from build123d import *

# Parameters (mm, degrees)
F0_W          = 17
F0_H          = 4
F1_DEPTH      = 50
F0_R          = 1.75
F0_R_2        = 11.5
F0_W_2        = 13
F2_DEPTH      = 3
F4_DEPTH      = 5
F4_DEPTH_BACK = 50
F6_DEPTH      = 3


with BuildPart() as f1:
    # F0 (on Top) → F1 (new body)
    with BuildSketch(Plane.XY):
        Polygon((-21.5, -21.5), (-21.5, 21.5), (-24.5, 21.5), (-24.5, -25.5), (-21.5, -25.5), align=None)
        Polygon((24.5, -25.5), (21.5, -25.5), (8.5, -25.5), (-8.5, -25.5), (-21.5, -25.5), (-24.5, -25.5), (-24.5, -28.5), (24.5, -28.5), align=None)
        Polygon((24.5, 21.5), (21.5, 21.5), (21.5, -21.5), (21.5, -25.5), (24.5, -25.5), align=None)
        with Locations((0, -23.5)):
            Rectangle(F0_W, F0_H)
    extrude(amount=F1_DEPTH)

    # F0 (on Top) → F2 (join)
    with BuildSketch(Plane.XY):
        Polygon((21.5, -21.5), (21.5, 21.5), (-21.5, 21.5), (-21.5, -21.5), (-8.5, -21.5), (8.5, -21.5), align=None)
        with Locations((-15.5, -15.5)):
            Circle(F0_R, mode=Mode.SUBTRACT)
        with Locations((15.5, -15.5)):
            Circle(F0_R, mode=Mode.SUBTRACT)
        Circle(F0_R_2, mode=Mode.SUBTRACT)
        with Locations((-15.5, 15.5)):
            Circle(F0_R, mode=Mode.SUBTRACT)
        with Locations((15.5, 15.5)):
            Circle(F0_R, mode=Mode.SUBTRACT)
        with Locations((15, -23.5)):
            Rectangle(F0_W_2, F0_H)
        with Locations((-15, -23.5)):
            Rectangle(F0_W_2, F0_H)
    extrude(amount=F2_DEPTH)

    # F3 (on face) → F4 (cut, two sides)
    with BuildSketch(Plane(origin=(21.5, 0, 0), x_dir=(0, -1, 0), z_dir=(-1, 0, 0))) as f4_sk:
        Polygon((-21.5, 3), (25.5, 50), (-21.5, 50), align=None)
    extrude(amount=-F4_DEPTH, mode=Mode.SUBTRACT)
    extrude(f4_sk.sketch, amount=F4_DEPTH_BACK, mode=Mode.SUBTRACT)

    # F5 (on face) → F6 (cut)
    with BuildSketch(Plane.XZ.offset(28.5)):
        with BuildLine():
            ThreePointArc((17.5943711698, 38.5), (17.1550313416, 39.5606601718), (16.0943711698, 40))
            Line((16.0943711698, 40), (15.5943711698, 40))
            ThreePointArc((15.5943711698, 40), (14.533710998, 39.5606601718), (14.0943711698, 38.5))
            Line((14.0943711698, 38.5), (14.0943711698, 11.5))
            ThreePointArc((14.0943711698, 11.5), (14.533710998, 10.4393398282), (15.5943711698, 10))
            Line((15.5943711698, 10), (16.0943711698, 10))
            ThreePointArc((16.0943711698, 10), (17.1550313416, 10.4393398282), (17.5943711698, 11.5))
            Line((17.5943711698, 11.5), (17.5943711698, 38.5))
        make_face()
        with BuildLine():
            Line((-13.4056288302, 11.5), (-13.4056288302, 38.5))
            ThreePointArc((-13.4056288302, 38.5), (-13.8449686584, 39.5606601718), (-14.9056288302, 40))
            Line((-14.9056288302, 40), (-15.4056288302, 40))
            ThreePointArc((-15.4056288302, 40), (-16.466289002, 39.5606601718), (-16.9056288302, 38.5))
            Line((-16.9056288302, 38.5), (-16.9056288302, 11.5))
            ThreePointArc((-16.9056288302, 11.5), (-16.466289002, 10.4393398282), (-15.4056288302, 10))
            Line((-15.4056288302, 10), (-14.9056288302, 10))
            ThreePointArc((-14.9056288302, 10), (-13.8449686584, 10.4393398282), (-13.4056288302, 11.5))
        make_face()
    extrude(amount=-F6_DEPTH, mode=Mode.SUBTRACT)


with BuildPart() as f7_1:
    # F7: copy of F1
    add(f1.part)


with BuildPart() as f9_1:
    # F9: copy of F1
    add(f1.part)


solid = f1.part
Geometry check sheet. Reference: the model listing, model coordinates, mm. A direction names the side the tool comes from. Give positions to 0.01 mm unless a question says otherwise; leave off trailing zeros. Write each loop counter-clockwise with the first axis right and the second up, starting at its lowest first coordinate (ties: lowest second). Pieces come first, ordered by that corner, then holes.
1) Go/stop test with flat-tipped pins: pin 1 Ø2 at (x, z) = (12.5, 38.5) entering from +Y; pin 2 Ø10.5 at (x, z) = (-12.5, 19.5) entering from +Y; pin 3 Ø1 at (x, y) = (-9.5, -18.5) entering from -Z; pin 4 Ø10 at (x, y) = (13, -1) entering from +Z. Record where each tip stops, or that it passes through.
Values follow:
pin 1: stops at y = -25.5
pin 2: stops at y = -21.5
pin 3: stops at z = 0
pin 4: stops at z = 3
2) Cross-section at B-B (x = 0). Record the boundary of the cut face in (y, z), plus the area to 3 significant figures.
Values follow:
outline: (-28.5, 0) - (-11.5, 0) - (-11.5, 3) - (-21.5, 3) - (-21.5, 46) - (-25.5, 50) - (-28.5, 50) - close; (11.5, 0) - (21.5, 0) - (21.5, 3) - (11.5, 3) - close
area: 402 mm2
3) Thickness scan on line 1 (X direction, y = -22.5, z = 6.5); line 2 (Y direction, x = -15.5, z = 2.3); line 3 (X direction, y = -15, z = 1). Record the ranges inside material, lowest first.
Values follow:
line 1: x = -24.5 to -21.5, -8.5 to 8.5, 21.5 to 24.5
line 2: y = -28.5 to -17.25, -13.75 to 13.75, 17.25 to 21.5
line 3: x = -24.5 to -17.18, -13.82 to 13.82, 17.18 to 24.5
4) Cross-section at A-A (z = 13). Record the boundary of the cut face in (x, y), plus the area to 3 significant figures.
Values follow:
outline: (-24.5, -28.5) - (-16.91, -28.5) - (-16.91, -25.5) - (-21.5, -25.5) - (-21.5, 11.5) - (-24.5, 11.5) - close; (-13.41, -28.5) - (14.09, -28.5) - (14.09, -25.5) - (8.5, -25.5) - (8.5, -21.5) - (-8.5, -21.5) - (-8.5, -25.5) - (-13.41, -25.5) - close; (17.59, -28.5) - (24.5, -28.5) - (24.5, 11.5) - (21.5, 11.5) - (21.5, -25.5) - (17.59, -25.5) - close
area: 416 mm2
5) Release check for a two-part mould opening along Z. For faces 1 (the face through (-13.857, -27.021, 10.428)), 2 (the face through (-16.455, -27.021, 39.572)), 3 (the face through (-21.5, -8, 21)), 4 (the face through (-23, -1.7, 26.2)) record: released by +Z, released by -Z, zero draft, split by the parting line, or undercut.
Values follow:
face 1: undercut
face 2: undercut
face 3: zero draft
face 4: released by +Z
6) Set-up check for faces 5 (the face through (-11.23, -3.15, 0)), 6 (the face through (0, -21.5, 24)), 7 (the face through (17.143, -27.021, 10.428)): record each of +Z, -Z, +X, -X, +Y, -Y from which the full face is reachable in a straight line by a thin tool's end or side.
Values follow:
face 5: -Z, +X, -X, +Y, -Y
face 6: +Z, +Y
face 7: +Y, -Y
7) Cross-section at D-D (y = 15.5). Record the boundary of the cut face in (x, z), plus the area to 3 significant figures.
Values follow:
outline: (-24.5, 0) - (-17.25, 0) - (-17.25, 3) - (-21.5, 3) - (-21.5, 9) - (-24.5, 9) - close; (-13.75, 0) - (13.75, 0) - (13.75, 3) - (-13.75, 3) - close; (17.25, 0) - (24.5, 0) - (24.5, 9) - (21.5, 9) - (21.5, 3) - (17.25, 3) - close
area: 162 mm2
8) Cross-section at C-C (y = 0). Record the boundary of the cut face in (x, z), plus the area to 3 significant figures.
Values follow:
outline: (-24.5, 0) - (-11.5, 0) - (-11.5, 3) - (-21.5, 3) - (-21.5, 24.5) - (-24.5, 24.5) - close; (11.5, 0) - (24.5, 0) - (24.5, 24.5) - (21.5, 24.5) - (21.5, 3) - (11.5, 3) - close
area: 207 mm2
